from build123d import *

# Parameters (mm, degrees)
F0_W     = 127
F0_H     = 127
F0_W_2   = 120.904
F0_H_2   = 120.904
F1_DEPTH = 1905
F3_DEPTH = 1905
F4_W     = 622.3
F4_H     = 6.35
F4_W_2   = 609.6
F5_DEPTH = 711.2
F6_W     = 1282.7
F6_H     = 177.8
F6_W_2   = 622.3
F7_DEPTH = 4.7625


with BuildPart() as f1:
    # F0 (on Right) → F1 (new body)
    with BuildSketch(Plane.YZ):
        with Locations((4.929526709, 15.0205540939)):
            Rectangle(F0_W, F0_H)
        with Locations((4.929526709, 15.0205540939)):
            Rectangle(F0_W_2, F0_H_2, mode=Mode.SUBTRACT)
    extrude(amount=F1_DEPTH)

    # F2 (on face) → F3 (join)
    with BuildSketch(Plane.YZ.offset(1905)):
        Polygon((-78.5117968917, 123.9730939269), (-58.570473291, 78.5205540939), (-53.4608645662, 78.5205540939), (-73.8704177914, 125.0403363069), align=None)
    extrude(amount=-F3_DEPTH)

    # F4 (on face) → F5 (join)
    with BuildSketch(Plane(origin=(0, 68.429526709, 0), x_dir=(-1, 0, 0), z_dir=(0, 1, 0))):
        with Locations((-311.15, -51.6544459061)):
            Rectangle(F4_W, F4_H)
        with Locations((-1104.9, -51.6544459061)):
            Rectangle(F4_W_2, F4_H)
    extrude(amount=-F5_DEPTH)

    # F6 (on face) → F7 (join)
    with BuildSketch(Plane.XY.offset(-48.4794459061)):
        with Locations((1263.65, -553.870473291)):
            Rectangle(F6_W, F6_H)
        with Locations((311.15, -553.870473291)):
            Rectangle(F6_W_2, F6_H)
    extrude(amount=F7_DEPTH)


solid = f1.part
Model file for the job. Use its own axes, mm. A direction names the side the tool comes from. Coordinates: 2 decimals unless noted, no trailing zeros. Order: outer loops, then holes, each group sorted by start corner. A loop starts at its lowest first (then second) coordinate and runs counter-clockwise, first axis right, second up. Notation, with made-up numbers: (29, 51) -> (50, 51) arc R19 cw to (50, 69) -> close; hole circle Ø2 at (89.25, 78). An arc over 180 degrees is marked (long way). Return JSON: item names as keys, results as strings. Group by question number.
Item 1: Saw through at C-C on x = 1638.5. Write the cut outline in (y, z), then the cut area to 3 significant figures.
Item 2: Saw through at B-B on y = -332. Write the cut outline in (x, z), then the cut area to 3 significant figures.
Item 3: Wall check: line 1 along Y through (x, z) = (206, 33); line 2 along Z through (x, y) = (1137, -313.5); line 3 along Z through (x, y) = (658, -566.5). Give the ranges that are in metal, low to high. Write a range as [from, to].
Item 4: Saw through at D-D on x = 492. Write the cut outline in (y, z), then the cut area to 3 significant figures.
Item 5: Pull direction Y, two halves, no side cores. Call faces 6 (the flat face through (939, 4, -45.431)), 7 (the flat face through (316, -282, -54.829)), 8 (the flat face through (965.84, -68.68, 101.56)), 9 (the flat face through (939, 65.382, 14)): pulls with the +Y half, pulls with the -Y half, needs draft (parallel to the pull), parting line crosses it, or undercut.
Item 6: Saw through at A-A on z = 18. Write the cut outline in (x, y).
Item 7: Flat gauge pins, fed straight in: P1, Ø1.9, axis at y = -165.5, z = -50.5, coming from the +X side; P2, Ø1.5, axis at x = 204.5, y = -571.5, coming from the +Z side; P3, Ø1.5, axis at x = 820.5, z = 42, coming from the -Y side. Where does each tip first touch, or does it go through?
Item 8: Tool access for faces 1 (the flat face through (939, 7, 78.521)), 2 (the flat face through (710, 4, -48.479)), 3 (the flat face through (939, -55.522, 14)), 4 (the flat face through (1654, 4, -48.479)), 5 (the flat face through (939, -553, -43.717)): list every direction of +Z, -Z, +X, -X, +Y, -Y with a clear straight run to the whole face (end or side of a thin tool).
Values found:
{
 "1": {"outline": "(-642.77, -48.48) -> (-464.97, -48.48) -> (-464.97, -43.72) -> (-642.77, -43.72) -> close; (-78.51, 123.97) -> (-58.57, 78.52) -> (-58.57, -48.48) -> (68.43, -48.48) -> (68.43, 78.52) -> (-53.46, 78.52) -> (-73.87, 125.04) -> close; hole (-55.52, -45.43) -> (65.38, -45.43) -> (65.38, 75.47) -> (-55.52, 75.47) -> close", "area": "2,590 mm2"},
 "2": {"outline": "(0, -54.83) -> (622.3, -54.83) -> (622.3, -48.48) -> (0, -48.48) -> close; (800.1, -54.83) -> (1409.7, -54.83) -> (1409.7, -48.48) -> (800.1, -48.48) -> close", "area": "7,820 mm2"},
 "3": {"line 1": "y = [-58.57, -55.52], [65.38, 68.43]", "line 2": "z = [-54.83, -48.48]", "line 3": "z = [-48.48, -43.72]"},
 "4": {"outline": "(-642.77, -54.83) -> (68.43, -54.83) -> (68.43, 78.52) -> (-53.46, 78.52) -> (-73.87, 125.04) -> (-78.51, 123.97) -> (-58.57, 78.52) -> (-58.57, -48.48) -> (-464.97, -48.48) -> (-464.97, -43.72) -> (-642.77, -43.72) -> close; hole (-55.52, -45.43) -> (65.38, -45.43) -> (65.38, 75.47) -> (-55.52, 75.47) -> close", "area": "7,110 mm2"},
 "5": {"face 6": "undercut", "face 7": "needs draft", "face 8": "pulls with the -Y half", "face 9": "undercut"},
 "6": {"outline": "(0, -58.57) -> (1905, -58.57) -> (1905, -55.52) -> (0, -55.52) -> close; (0, 65.38) -> (1905, 65.38) -> (1905, 68.43) -> (0, 68.43) -> close"},
 "7": {"P1": "stops at x = 1409.7", "P2": "stops at z = -43.72", "P3": "stops at y = -58.57"},
 "8": {"face 1": "+Z, +X, -X, +Y", "face 2": "-Z, +Y, -Y", "face 3": "+X, -X", "face 4": "-Z, +X, +Y, -Y", "face 5": "+Z, +X, -X, -Y"}
}
